Build history of the part. All positions in model axes, mm. Face numbers are marked on the shaded views. Round coordinates to 2 decimals unless told otherwise and drop trailing zeros. Order: outer loops, then holes, each group sorted by start corner. A loop starts at its lowest first (then second) coordinate and runs counter-clockwise, first axis right, second up. Notation, with made-up numbers: (52, -36) -> (93, -36) arc R27 ccw to (93, 1) -> close; hole circle Ø6 at (25, -19). An arc over 180 degrees is marked (long way). Use a Markdown table: item, result. Add a question column.
Item 1: Pin check, flat tips, straight feed: pin 1 (4 mm diameter, centred on x = -32.79, y = -436.56, fed in from +Z); pin 2 (6 mm diameter, centred on y = -387.5, z = 44.5, fed in from +X). Stop position of each tip, or through.
Item 2: Slice it at C-C, the plane z = 48. Give the cut face in (x, y), plus the area to 3 significant figures.
Item 3: Slice it at A-A, the plane x = -23.5. Give the cut face in (y, z), plus the area to 3 significant figures.
Item 4: Slice it at B-B, the plane y = -320. Give the cut face in (x, z).
Item 5: Probe L1, parallel to Z at x = -39, y = -168; L2, parallel to X at y = -435, z = 42.5; L3, parallel to Z at x = -5.5, y = -269. List the from-to ranges inside material, lowest first.
Item 6: Two-plate mould, pull along Z, no slides. Class the marked faces 1 and 2: released by +Z, released by -Z, zero draft, split by the parting line, or undercut.
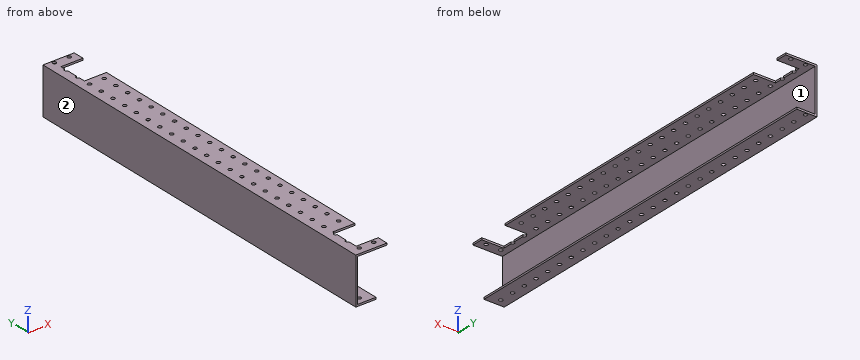
from build123d import *

# Parameters (mm, degrees)
F1_DEPTH = 677.8625
F2_W     = 38.1
F2_H     = 50.8
F3_DEPTH = 25.4
F4_R     = 3.175
F5_DEPTH = 101.6


with BuildPart() as f1:
    # F0 (on Front) → F1 (new body)
    with BuildSketch(Plane.XZ):
        Polygon((5.314447, 57.120183), (-48.660553, 57.120183), (-48.660553, -23.270817), (-13.735553, -23.270817), (-13.735553, -20.095817), (-45.485553, -20.095817), (-45.485553, 53.945183), (5.314447, 53.945183), align=None)
    extrude(amount=F1_DEPTH)

    # F2 (on face) → F3 (cut)
    with BuildSketch(Plane(origin=(0, 0, 53.945183), x_dir=(1, 0, 0), z_dir=(0, 0, -1))):
        with Locations((-13.735553, 44.45)):
            Rectangle(F2_W, F2_H)
        with Locations((-13.735553, 633.4125)):
            Rectangle(F2_W, F2_H)
    extrude(amount=-F3_DEPTH, mode=Mode.SUBTRACT)

    # F4 (on face) → F5 (cut)
    with BuildSketch(Plane.XY.offset(57.120183)):
        with Locations((-7.385553, -665.1625)):
            Circle(F4_R)
        with Locations((-7.385553, -639.7625)):
            Circle(F4_R)
        with Locations((-7.385553, -614.3625)):
            Circle(F4_R)
        with Locations((-7.385553, -588.9625)):
            Circle(F4_R)
        with Locations((-7.385553, -563.5625)):
            Circle(F4_R)
        with Locations((-7.385553, -538.1625)):
            Circle(F4_R)
        with Locations((-7.385553, -512.7625)):
            Circle(F4_R)
        with Locations((-7.385553, -487.3625)):
            Circle(F4_R)
        with Locations((-7.385553, -461.9625)):
            Circle(F4_R)
        with Locations((-7.385553, -436.5625)):
            Circle(F4_R)
        with Locations((-7.385553, -411.1625)):
            Circle(F4_R)
        with Locations((-7.385553, -385.7625)):
            Circle(F4_R)
        with Locations((-7.385553, -360.3625)):
            Circle(F4_R)
        with Locations((-7.385553, -334.9625)):
            Circle(F4_R)
        with Locations((-7.385553, -309.5625)):
            Circle(F4_R)
        with Locations((-7.385553, -284.1625)):
            Circle(F4_R)
        with Locations((-7.385553, -258.7625)):
            Circle(F4_R)
        with Locations((-7.385553, -233.3625)):
            Circle(F4_R)
        with Locations((-7.385553, -207.9625)):
            Circle(F4_R)
        with Locations((-7.385553, -182.5625)):
            Circle(F4_R)
        with Locations((-7.385553, -157.1625)):
            Circle(F4_R)
        with Locations((-7.385553, -131.7625)):
            Circle(F4_R)
        with Locations((-7.385553, -106.3625)):
            Circle(F4_R)
        with Locations((-7.385553, -80.9625)):
            Circle(F4_R)
        with Locations((-7.385553, -55.5625)):
            Circle(F4_R)
        with Locations((-7.385553, -30.1625)):
            Circle(F4_R)
        with Locations((-7.385553, -4.7625)):
            Circle(F4_R)
        with Locations((-32.785553, -665.1625)):
            Circle(F4_R)
        with Locations((-32.785553, -639.7625)):
            Circle(F4_R)
        with Locations((-32.785553, -614.3625)):
            Circle(F4_R)
        with Locations((-32.785553, -588.9625)):
            Circle(F4_R)
        with Locations((-32.785553, -563.5625)):
            Circle(F4_R)
        with Locations((-32.785553, -538.1625)):
            Circle(F4_R)
        with Locations((-32.785553, -512.7625)):
            Circle(F4_R)
        with Locations((-32.785553, -487.3625)):
            Circle(F4_R)
        with Locations((-32.785553, -461.9625)):
            Circle(F4_R)
        with Locations((-32.785553, -436.5625)):
            Circle(F4_R)
        with Locations((-32.785553, -411.1625)):
            Circle(F4_R)
        with Locations((-32.785553, -385.7625)):
            Circle(F4_R)
        with Locations((-32.785553, -360.3625)):
            Circle(F4_R)
        with Locations((-32.785553, -334.9625)):
            Circle(F4_R)
        with Locations((-32.785553, -309.5625)):
            Circle(F4_R)
        with Locations((-32.785553, -284.1625)):
            Circle(F4_R)
        with Locations((-32.785553, -258.7625)):
            Circle(F4_R)
        with Locations((-32.785553, -233.3625)):
            Circle(F4_R)
        with Locations((-32.785553, -207.9625)):
            Circle(F4_R)
        with Locations((-32.785553, -182.5625)):
            Circle(F4_R)
        with Locations((-32.785553, -157.1625)):
            Circle(F4_R)
        with Locations((-32.785553, -131.7625)):
            Circle(F4_R)
        with Locations((-32.785553, -106.3625)):
            Circle(F4_R)
        with Locations((-32.785553, -80.9625)):
            Circle(F4_R)
        with Locations((-32.785553, -55.5625)):
            Circle(F4_R)
        with Locations((-32.785553, -30.1625)):
            Circle(F4_R)
        with Locations((-32.785553, -4.7625)):
            Circle(F4_R)
    extrude(amount=-F5_DEPTH, mode=Mode.SUBTRACT)


solid = f1.part
Check sheet entries:
| question | item | result |
|---|---|---|
| 1 | pin 1 | through |
| 1 | pin 2 | x = -45.49 |
| 2 | outline | (-48.66, -677.86) -> (-45.49, -677.86) -> (-45.49, 0) -> (-48.66, 0) -> close |
| 2 | area | 2,150 mm2 |
| 3 | outline | (-677.86, -23.27) -> (0, -23.27) -> (0, -20.1) -> (-677.86, -20.1) -> close; (-677.86, 53.95) -> (-658.81, 53.95) -> (-658.81, 57.12) -> (-677.86, 57.12) -> close; (-608.01, 53.95) -> (-69.85, 53.95) -> (-69.85, 57.12) -> (-608.01, 57.12) -> close; (-19.05, 53.95) -> (0, 53.95) -> (0, 57.12) -> (-19.05, 57.12) -> close |
| 3 | area | 3,980 mm2 |
| 4 | outline | (-48.66, -23.27) -> (-13.74, -23.27) -> (-13.74, -20.1) -> (-45.49, -20.1) -> (-45.49, 53.95) -> (5.31, 53.95) -> (5.31, 57.12) -> (-48.66, 57.12) -> close |
| 5 | L1 | -23.27 to -20.1, 53.95 to 57.12 |
| 5 | L2 | -48.66 to -45.49 |
| 5 | L3 | 53.95 to 57.12 |
| 6 | face 1 | undercut |
| 6 | face 2 | zero draft |
